from build123d import *

# Parameters (mm, degrees)
SKETCH1_W                                      = 2
SKETCH1_H                                      = 7.5
SKETCH1_W_2                                    = 10
SKETCH1_W_3                                    = 5.5
SKETCH1_W_4                                    = 17.49
SKETCH1_H_2                                    = 5.375
SKETCH1_R                                      = 1.75
BOSS_EXTRUDE1_DEPTH                            = 1.5
BOSS_EXTRUDE2_START                            = -4
SKETCH1_4_R                                    = 1.75
SKETCH1_4_W                                    = 2
SKETCH1_4_H                                    = 7.5
BOSS_EXTRUDE2_DEPTH                            = 4
CSK_FOR_M2_FLAT_HEAD_MACHINE_SCREW1_AT_2_COUNT = 2
CSK_FOR_M2_FLAT_HEAD_MACHINE_SCREW1_AT_2_PITCH = 22.4144
CSK_FOR_M2_FLAT_HEAD_MACHINE_SCREW1_AT_3_COUNT = 2
CSK_FOR_M2_FLAT_HEAD_MACHINE_SCREW1_AT_3_PITCH = 22.4144
FILLET1_R                                      = 1


with BuildPart() as part:
    # Sketch1 → Boss-Extrude1 (new body)
    # profile 1 of 10: a face of its own
    with BuildSketch(Plane(origin=(0, 0, 0), x_dir=(1, 0, 0), z_dir=(0, 1, 0))):
        with Locations((13.75, 0)):
            Rectangle(SKETCH1_W, SKETCH1_H)
    # profile 2 of 10: a face of its own
    with BuildSketch(Plane(origin=(0, 0, 0), x_dir=(1, 0, 0), z_dir=(0, 1, 0))):
        with Locations((7.75, 0)):
            Rectangle(SKETCH1_W_2, SKETCH1_H)
    # profile 3 of 10: a face of its own
    with BuildSketch(Plane(origin=(0, 0, 0), x_dir=(1, 0, 0), z_dir=(0, 1, 0))):
        Rectangle(SKETCH1_W_3, SKETCH1_H)
    # profile 4 of 10: a face of its own
    with BuildSketch(Plane(origin=(0, 0, 0), x_dir=(1, 0, 0), z_dir=(0, 1, 0))):
        with Locations((-11.495, 0)):
            Rectangle(SKETCH1_W_4, SKETCH1_H)
    # profile 5 of 10: a face of its own
    with BuildSketch(Plane(origin=(0, 0, 0), x_dir=(1, 0, 0), z_dir=(0, 1, 0))):
        with Locations((0, -6.4375)):
            Rectangle(SKETCH1_W_3, SKETCH1_H_2)
    # profile 6 of 10: a face of its own
    with BuildSketch(Plane(origin=(0, 0, 0), x_dir=(1, 0, 0), z_dir=(0, 1, 0))):
        with Locations((0, 6.4375)):
            Rectangle(SKETCH1_W_3, SKETCH1_H_2)
    # profile 7 of 10: a face of its own
    with BuildSketch(Plane(origin=(0, 0, 0), x_dir=(1, 0, 0), z_dir=(0, 1, 0))):
        with BuildLine():
            Line((2.75, 9.125), (2.75, 11.2072))
            ThreePointArc((2.75, 11.2072), (0, 13.9572), (-2.75, 11.2072))
            Line((-2.75, 11.2072), (-2.75, 9.125))
            Line((-2.75, 9.125), (2.75, 9.125))
        make_face()
        with Locations((0, 11.2072)):
            Circle(SKETCH1_R, mode=Mode.SUBTRACT)
    # profile 8 of 10: a face of its own
    with BuildSketch(Plane(origin=(0, 0, 0), x_dir=(1, 0, 0), z_dir=(0, 1, 0))):
        with Locations((0, 11.2072)):
            Circle(SKETCH1_R)
    # profile 9 of 10: a face of its own
    with BuildSketch(Plane(origin=(0, 0, 0), x_dir=(1, 0, 0), z_dir=(0, 1, 0))):
        with BuildLine():
            Line((2.75, -11.2072), (2.75, -9.125))
            Line((2.75, -9.125), (-2.75, -9.125))
            Line((-2.75, -9.125), (-2.75, -11.2072))
            ThreePointArc((-2.75, -11.2072), (0, -13.9572), (2.75, -11.2072))
        make_face()
        with Locations((0, -11.2072)):
            Circle(SKETCH1_R, mode=Mode.SUBTRACT)
    # profile 10 of 10: a face of its own
    with BuildSketch(Plane(origin=(0, 0, 0), x_dir=(1, 0, 0), z_dir=(0, 1, 0))):
        with Locations((0, -11.2072)):
            Circle(SKETCH1_R)
    extrude(amount=BOSS_EXTRUDE1_DEPTH)

    # Sketch1_4 → Boss-Extrude2 (add)
    # profile 1 of 5: a face of its own
    with BuildSketch(Plane(origin=(0, 0, 0), x_dir=(1, 0, 0), z_dir=(0, 1, 0)).offset(BOSS_EXTRUDE2_START)):
        with BuildLine():
            Line((2.75, 9.125), (2.75, 11.2072))
            ThreePointArc((2.75, 11.2072), (0, 13.9572), (-2.75, 11.2072))
            Line((-2.75, 11.2072), (-2.75, 9.125))
            Line((-2.75, 9.125), (2.75, 9.125))
        make_face()
        with Locations((0, 11.2072)):
            Circle(SKETCH1_4_R, mode=Mode.SUBTRACT)
    # profile 2 of 5: a face of its own
    with BuildSketch(Plane(origin=(0, 0, 0), x_dir=(1, 0, 0), z_dir=(0, 1, 0)).offset(BOSS_EXTRUDE2_START)):
        with BuildLine():
            Line((2.75, -11.2072), (2.75, -9.125))
            Line((2.75, -9.125), (-2.75, -9.125))
            Line((-2.75, -9.125), (-2.75, -11.2072))
            ThreePointArc((-2.75, -11.2072), (0, -13.9572), (2.75, -11.2072))
        make_face()
        with Locations((0, -11.2072)):
            Circle(SKETCH1_4_R, mode=Mode.SUBTRACT)
    # profile 3 of 5: a face of its own
    with BuildSketch(Plane(origin=(0, 0, 0), x_dir=(1, 0, 0), z_dir=(0, 1, 0)).offset(BOSS_EXTRUDE2_START)):
        with Locations((13.75, 0)):
            Rectangle(SKETCH1_4_W, SKETCH1_4_H)
    # profile 4 of 5: a face of its own
    with BuildSketch(Plane(origin=(0, 0, 0), x_dir=(1, 0, 0), z_dir=(0, 1, 0)).offset(BOSS_EXTRUDE2_START)):
        with Locations((0, 11.2072)):
            Circle(SKETCH1_4_R)
    # profile 5 of 5: a face of its own
    with BuildSketch(Plane(origin=(0, 0, 0), x_dir=(1, 0, 0), z_dir=(0, 1, 0)).offset(BOSS_EXTRUDE2_START)):
        with Locations((0, -11.2072)):
            Circle(SKETCH1_4_R)
    extrude(amount=BOSS_EXTRUDE2_DEPTH)

    # Sketch3 → CSK for M2 Flat Head Machine Screw1 (revolve, cut)
    with BuildSketch(Plane(origin=(0, 1.5, 11.2072), x_dir=(0, 0, 1), z_dir=(1, 0, 0))):
        Polygon((0, 0), (0, 5.5), (1.2, 5.5), (1.2, 1), (2.2, 0), align=None)
    csk_for_m2_flat_head_machine_screw1 = revolve(axis=Axis((0, 7.85, 11.2072), (0, -1, 0)), mode=Mode.SUBTRACT)

    # CSK for M2 Flat Head Machine Screw1 at 2: CSK for M2 Flat Head Machine Screw1 ×2
    with Locations(*[(0, 0, -i * CSK_FOR_M2_FLAT_HEAD_MACHINE_SCREW1_AT_2_PITCH) for i in range(1, CSK_FOR_M2_FLAT_HEAD_MACHINE_SCREW1_AT_2_COUNT)]):
        add(csk_for_m2_flat_head_machine_screw1, mode=Mode.SUBTRACT)

    # CSK for M2 Flat Head Machine Screw1 at 3: CSK for M2 Flat Head Machine Screw1 ×2
    with Locations(*[(0, 0, -i * CSK_FOR_M2_FLAT_HEAD_MACHINE_SCREW1_AT_3_PITCH) for i in range(1, CSK_FOR_M2_FLAT_HEAD_MACHINE_SCREW1_AT_3_COUNT)]):
        add(csk_for_m2_flat_head_machine_screw1, mode=Mode.SUBTRACT)

    # Fillet1
    fillet1_edges = [part.edges().sort_by_distance(p)[0] for p in [
        (14.75, -1.25, 3.75),
        (2.75, 0.75, 3.75),
        (-2.75, 0.75, 3.75),
        (-20.24, 0.75, 3.75),
        (-20.24, 0.75, -3.75),
        (-2.75, 0.75, -3.75),
        (2.75, 0.75, -3.75),
        (14.75, -1.25, -3.75),
    ]]
    fillet(fillet1_edges, radius=FILLET1_R)


solid = part.part
Read the model definition and answer for the solid it produces. Units are mm, in the model's axes. A direction names the side the tool comes from. Round coordinates to 2 decimals unless told otherwise and drop trailing zeros. Loops run counter-clockwise (first coordinate to the right, second up) from the corner with the lowest first, then second, coordinate; pieces in that order, holes last.
Q1. Each of these flat-tipped pins is pushed along its axis until it touches: pin 1 (1.2 mm diameter, centred on x = 1, y = -2, fed in from +Z); pin 2 (1 mm diameter, centred on x = 7, z = -3.5, fed in from -Y); pin 3 (1.2 mm diameter, centred on y = -2, z = -0.5, fed in from -X). Where does it stop, or does it pass through?
Q2. Section C-C on y = 1.1 is taken. Write down the section's boundary in (x, z).
Q3. Section A-A on y = -1.2 is taken. Write down the section's boundary in (x, z) (3 decimals).
Q4. Determine the mould class of faces 5 (the face through (0, -2, 9.125)), 6 (the face through (14.449, -1.212, 3.465)), 7 (the face through (-20.24, 1, 0)) for opening direction Z: released by +Z, released by -Z, zero draft, split by the parting line, or undercut.
Q5. Which of the six approach directions +Z, -Z, +X, -X, +Y, -Y give full straight-line access (tool end or side, diameter ignored) to faces 1 (the face through (-2.75, -0.7, 9.4)), 2 (the face through (12.75, -2, 0)), 3 (the face through (9.8, 0.4, -3.75)), 4 (the face through (9.8, 0.4, 3.75))?
Q6. Section D-D on x = 5 is taken. Write down the section's boundary in (y, z), and give its area (4 significant figures).
Q7. Section B-B on x = 0 is taken. Write down the section's boundary in (y, z) (3 decimals), and give its area (3 significant figures).
Q8. Consider probe 1 along Z at (x, y) = (0, -1.8) (3 decimals); probe 2 along Z at (x, y) = (1.5, -1.95) (3 decimals); probe 3 along Z at (x, y) = (2, -1.3) (3 decimals). Determine where each line is inside the solid, lowest interval first.
Output:
1. pin 1: stops at z = 13.93
1. pin 2: stops at y = 0
1. pin 3: stops at x = 12.75
2. outline: (-20.24, -2.75) arc R1 ccw to (-19.24, -3.75) - (-3.75, -3.75) arc R1 cw to (-2.75, -4.75) - (-2.75, -11.21) arc R2.75 ccw to (2.75, -11.21) - (2.75, -4.75) arc R1 cw to (3.75, -3.75) - (13.75, -3.75) arc R1 ccw to (14.75, -2.75) - (14.75, 2.75) arc R1 ccw to (13.75, 3.75) - (3.75, 3.75) arc R1 cw to (2.75, 4.75) - (2.75, 11.21) arc R2.75 ccw to (-2.75, 11.21) - (-2.75, 4.75) arc R1 cw to (-3.75, 3.75) - (-19.24, 3.75) arc R1 ccw to (-20.24, 2.75) - close; hole circle Ø3.6 at (0, -11.21); hole circle Ø3.6 at (0, 11.21)
3. outline: (-2.75, -11.207) arc R2.75 ccw to (2.75, -11.207) - (2.75, -9.125) - (-2.75, -9.125) - close; (-2.75, 9.125) - (2.75, 9.125) - (2.75, 11.207) arc R2.75 ccw to (-2.75, 11.207) - close; (12.75, -3.75) - (13.75, -3.75) arc R1 ccw to (14.75, -2.75) - (14.75, 2.75) arc R1 ccw to (13.75, 3.75) - (12.75, 3.75) - close; hole circle Ø2.4 at (0, -11.207); hole circle Ø2.4 at (0, 11.207)
4. face 5: undercut
4. face 6: released by +Z
4. face 7: zero draft
5. face 1: +Z, -X, +Y, -Y
5. face 2: +Z, -Z, -X, -Y
5. face 3: -Z, +X, +Y, -Y
5. face 4: +Z, +X, +Y, -Y
6. outline: (0, -3.75) - (1.5, -3.75) - (1.5, 3.75) - (0, 3.75) - close
6. area: 11.25 mm2
7. outline: (-4, -13.957) - (1.5, -13.957) - (1.5, -13.407) - (0.5, -12.407) - (-4, -12.407) - close; (-4, -10.007) - (0.5, -10.007) - (1.5, -9.007) - (1.5, 9.007) - (0.5, 10.007) - (-4, 10.007) - (-4, 9.125) - (0, 9.125) - (0, -9.125) - (-4, -9.125) - close; (-4, 12.407) - (0.5, 12.407) - (1.5, 13.407) - (1.5, 13.957) - (-4, 13.957) - close
7. area: 52.1 mm2
8. probe 1: z = -13.957 to -12.407, -10.007 to -9.125, 9.125 to 10.007, 12.407 to 13.957
8. probe 2: z = -13.512 to -9.125, 9.125 to 13.512
8. probe 3: z = -13.095 to -9.125, 9.125 to 13.095
